```python
from build123d import *

# Parameters (mm, degrees)
BOSS_EXTRUDE1_DEPTH = 70
FILLET1_R           = 10
FILLET2_R           = 10
SKETCH2_R           = 12.5
CUT_EXTRUDE1_DEPTH  = 86


with BuildPart() as part:
    # Sketch1 → Boss-Extrude1 (new body)
    with BuildSketch(Plane.XY):
        Polygon((0, 62), (0, 52), (75.857864376, 52), (102.857864376, 25), (0, 25), (0, 0), (710, 0), (710, 25), (626.905989232, 25), (655.773502692, 75), (710, 75), (710, 85), (650, 85), (622.287187079, 37), (570, 37), (570, 25), (180, 25), (180, 37), (105, 37), (80, 62), align=None)
    extrude(amount=BOSS_EXTRUDE1_DEPTH)

    # Fillet1
    fillet1_edges = [part.edges().sort_by_distance(p)[0] for p in [
        (80, 62, 35),
        (105, 37, 35),
        (650, 85, 35),
        (622.287187079, 37, 35),
    ]]
    fillet(fillet1_edges, radius=FILLET1_R)

    # Fillet2
    fillet2_edges = [part.edges().sort_by_distance(p)[0] for p in [
        (75.857864376, 52, 35),
        (655.773502692, 75, 35),
    ]]
    fillet(fillet2_edges, radius=FILLET2_R)

    # Sketch2 → Cut-Extrude1 (cut, through all)
    with BuildSketch(Plane(origin=(0, 85, 0), x_dir=(1, 0, 0), z_dir=(0, 1, 0))):
        with Locations((680, -35)):
            Circle(SKETCH2_R)
        with Locations((30, -35)):
            Circle(SKETCH2_R)
    extrude(amount=-CUT_EXTRUDE1_DEPTH, mode=Mode.SUBTRACT)


solid = part.part
```
Build history of the part. All positions in model axes, mm. A direction names the side the tool comes from. Give positions to 0.01 mm unless a question says otherwise; leave off trailing zeros. Order: outer loops, then holes, each group sorted by start corner. A loop starts at its lowest first (then second) coordinate and runs counter-clockwise, first axis right, second up. Notation, with made-up numbers: M -11,-22.75 L 7,-22.75 A33 ccw 7,8.25 Z; hole C 6,66.5 d8. An arc over 180 degrees is marked long. Return JSON: item names as keys, results as strings.
Q1. Two-plate mould, pull along Z, no slides. Class faces 4 (the face through (350, 24, 0)), 5 (the face through (710, 12, 35)), 6 (the face through (20.79, 57.07, 26.55)): pulls with the +Z half, pulls with the -Z half, needs draft (parallel to the pull), parting line crosses it, or undercut.
Answer list:
{"face 4": "pulls with the -Z half", "face 5": "needs draft", "face 6": "undercut"}
Q2. Band-saw the part on A-A (x = 30). Give the cut face in (y, z).
Answer list:
{"outline": "M 0,0 L 25,0 L 25,22.5 L 0,22.5 Z; M 0,47.5 L 25,47.5 L 25,70 L 0,70 Z; M 52,0 L 62,0 L 62,22.5 L 52,22.5 Z; M 52,47.5 L 62,47.5 L 62,70 L 52,70 Z"}
Q3. Flat gauge pins, fed straight in: pin 1 (21 mm diameter, centred on x = 54.5, z = 34, fed in from +Y); pin 2 (2 mm diameter, centred on y = 42, z = 35.5, fed in from +X); pin 3 (3.5 mm diameter, centred on y = 33.5, z = 18, fed in from -X). Where does each tip first touch, or does it go through?
Answer list:
{"pin 1": "stops at y = 62", "pin 2": "stops at x = 637.3", "pin 3": "stops at x = 92.61"}
Q4. Band-saw the part on D-D (x = 485.5). Give the cut face in (y, z), then the cut area to 3 significant figures.
Answer list:
{"outline": "M 0,0 L 25,0 L 25,70 L 0,70 Z", "area": "1,750 mm^2"}
Q5. 3-axis set-ups, long thin cutter, end or side, ignore diameter. For faces 1 (the face through (47, 62, 35)), 2 (the face through (669, 25, 42)), 3 (the face through (636.3, 61.27, 34.51)): which of +Z, -Z, +X, -X, +Y, -Y reach the whole face in a straight line?
Answer list:
{"face 1": "+Z, -Z, -X, +Y", "face 2": "+Z, -Z, +X", "face 3": "+Z, -Z, +Y"}
Q6. Band-saw the part on C-C (z = 35). Count the separate pieces of the cut face and the enclosed holes in it, then the cut area to 3 significant figures.
Answer list:
{"separate pieces": "5", "enclosed holes": "0", "area": "19,900 mm^2"}
Q7. Wall check: probe 1 along X at (y, z) = (17, 35); probe 2 along Z at (x, y) = (30, 58); probe 3 along X at (y, z) = (58.5, 35). Give the ranges that are in metal, low to high. Write a range as from..to.
Answer list:
{"probe 1": "x = 0..17.5, 42.5..667.5, 692.5..710", "probe 2": "z = 0..22.5, 47.5..70", "probe 3": "x = 0..17.5, 42.5..83.5, 634.7..646.25"}
Q8. Band-saw the part on B-B (y = 7.5). Give the cut face in (x, z), then the cut area to 3 significant figures.
Answer list:
{"outline": "M 0,0 L 710,0 L 710,70 L 0,70 Z; hole C 30,35 d25; hole C 680,35 d25", "area": "48,700 mm^2"}
